```python
from build123d import *

# Parameters (mm, degrees)
SKETCH1_W             = 180
SKETCH1_H             = 180
BOSS_EXTRUDE1_DEPTH   = 3
FILLET1_R             = 15
SKETCH2_R             = 1.6
SKETCH2_W             = 25
SKETCH2_H             = 90
CUT_EXTRUDE2_DEPTH    = 128.314571044
FILLET2_R             = 10
HOLE_WIZARD_3_0_3_1_D = 3
HOLE_WIZARD_3_0_3_2_D = 3
HOLE_WIZARD_4_0_4_1_D = 4
SKETCH3_R             = 1.5
SKETCH3_R_2           = 1.6
CUT_EXTRUDE3_DEPTH    = 128.314571044
SKETCH4_R             = 1.5
CUT_EXTRUDE4_DEPTH    = 128.314571044
SKETCH5_R             = 12.5
CUT_EXTRUDE5_DEPTH    = 128.314571044
FILLET3_R             = 2


with BuildPart() as part:
    # Sketch1 → Boss-Extrude1 (new body)
    with BuildSketch(Plane(origin=(0, 0, 0), x_dir=(1, 0, 0), z_dir=(0, 1, 0))):
        Rectangle(SKETCH1_W, SKETCH1_H)
    extrude(amount=BOSS_EXTRUDE1_DEPTH)

    # Fillet1
    fillet1_edges = [part.edges().sort_by_distance(p)[0] for p in [
        (90, 1.5, 90),
        (-90, 1.5, 90),
        (-90, 1.5, -90),
        (90, 1.5, -90),
    ]]
    fillet(fillet1_edges, radius=FILLET1_R)

    # Sketch2 → Cut-Extrude2 (cut, through all)
    with BuildSketch(Plane(origin=(0, 3, 0), x_dir=(1, 0, 0), z_dir=(0, 1, 0))):
        with Locations(Location((-60.05, 20, 0), (0, 0, 270))):
            Circle(SKETCH2_R)
        with Locations(Location((-49.05, 20, 0), (0, 0, 270))):
            Circle(SKETCH2_R)
        with Locations(Location((-60.05, -20, 0), (0, 0, 270))):
            Circle(SKETCH2_R)
        with Locations(Location((-49.05, -20, 0), (0, 0, 270))):
            Circle(SKETCH2_R)
        with Locations(Location((49.05, 20, 0), (0, 0, 270))):
            Circle(SKETCH2_R)
        with Locations(Location((60.05, 20, 0), (0, 0, 270))):
            Circle(SKETCH2_R)
        with Locations(Location((49.05, -20, 0), (0, 0, 270))):
            Circle(SKETCH2_R)
        with Locations(Location((60.05, -20, 0), (0, 0, 270))):
            Circle(SKETCH2_R)
        with Locations((-77.5, 0)):
            Rectangle(SKETCH2_W, SKETCH2_H)
        with Locations((77.5, 0)):
            Rectangle(SKETCH2_W, SKETCH2_H)
    extrude(amount=-CUT_EXTRUDE2_DEPTH, mode=Mode.SUBTRACT)

    # Fillet2
    fillet2_edges = [part.edges().sort_by_distance(p)[0] for p in [
        (-65, 1.5, -45),
        (-65, 1.5, 45),
        (-90, 1.5, 45),
        (-90, 1.5, -45),
        (90, 1.5, -45),
        (90, 1.5, 45),
        (65, 1.5, 45),
        (65, 1.5, -45),
    ]]
    fillet(fillet2_edges, radius=FILLET2_R)

    # Диаметр отверстия Ø3.0 (3)1 (through all)
    with Locations(Plane(origin=(0, 3, 0), x_dir=(1, 0, 0), z_dir=(0, 1, 0))):
        with Locations((-65, -65), (-65, 65), (65, 65), (65, -65)):
            Hole(HOLE_WIZARD_3_0_3_1_D / 2)

    # Диаметр отверстия Ø3.0 (3)2 (through all)
    with Locations(Plane(origin=(0, 3, 0), x_dir=(1, 0, 0), z_dir=(0, 1, 0))):
        with Locations((-5, 15), (-38.5, 45.5), (-38.5, 55.5), (5, 15), (38.5, 45.5), (38.5, 55.5), (5, 86), (-5, 86)):
            Hole(HOLE_WIZARD_3_0_3_2_D / 2)

    # Диаметр отверстия Ø4.0 (4)1 (through all)
    with Locations(Plane(origin=(0, 3, 0), x_dir=(1, 0, 0), z_dir=(0, 1, 0))):
        with Locations((-19.5, 60), (19.5, 60)):
            Hole(HOLE_WIZARD_4_0_4_1_D / 2)

    # Sketch3 → Cut-Extrude3 (cut, through all)
    with BuildSketch(Plane(origin=(0, 3, 0), x_dir=(1, 0, 0), z_dir=(0, 1, 0))):
        with Locations(Location((-6, -72, 0), (0, 0, 270))):
            Circle(SKETCH3_R)
        with Locations(Location((6, -72, 0), (0, 0, 90))):
            Circle(SKETCH3_R)
        with Locations(Location((53.371589587, -44.65, 0), (0, 0, 270))):
            Circle(SKETCH3_R_2)
        with Locations(Location((-53.371589587, -44.65, 0), (0, 0, 270))):
            Circle(SKETCH3_R_2)
    extrude(amount=-CUT_EXTRUDE3_DEPTH, mode=Mode.SUBTRACT)

    # Sketch4 → Cut-Extrude4 (cut, through all)
    with BuildSketch(Plane(origin=(0, 3, 0), x_dir=(1, 0, 0), z_dir=(0, 1, 0))):
        with Locations(Location((-36, 83.5, 0), (0, 0, 270))):
            Circle(SKETCH4_R)
        with Locations(Location((37, 83.5, 0), (0, 0, 270))):
            Circle(SKETCH4_R)
        with Locations(Location((37, 26.5, 0), (0, 0, 270))):
            Circle(SKETCH4_R)
        with Locations(Location((-36, 26.5, 0), (0, 0, 270))):
            Circle(SKETCH4_R)
    extrude(amount=-CUT_EXTRUDE4_DEPTH, mode=Mode.SUBTRACT)

    # Sketch5 → Cut-Extrude5 (cut, through all)
    with BuildSketch(Plane(origin=(0, 3, 0), x_dir=(1, 0, 0), z_dir=(0, 1, 0))):
        with Locations(Location((0, 60, 0), (0, 0, 270))):
            Circle(SKETCH5_R)
        Polygon((31.754264805, 5), (0, -50), (-31.754264805, 5), (-24.826061575, 9), (0, -34), (24.826061575, 9), align=None)
        Polygon((0, -18), (15.588457268, 9), (-15.588457268, 9), align=None)
        Polygon((-5, -57.339745962), (-23.392304845, -57.339745962), (-45.598076211, -44.519237886), (-29, -15.770526581), align=None)
        Polygon((29, -15.770526581), (5, -57.339745962), (23.392304845, -57.339745962), (45.598076211, -44.519237886), align=None)
        with BuildLine():
            Line((-14.800549998, 50.996092632), (-27.5, 29))
            Line((-27.5, 29), (27.5, 29))
            Line((27.5, 29), (14.800549998, 50.996092632))
            Line((14.800549998, 50.996092632), (9.435897436, 47.078551181))
            ThreePointArc((9.435897436, 47.078551181), (0, 44), (-9.435897436, 47.078551181))
            Line((-9.435897436, 47.078551181), (-14.800549998, 50.996092632))
        make_face()
        Polygon((-59, -57.56624327), (-26.725386608, -76.2), (-59, -76.2), align=None)
        Polygon((-49.007586221, 49.3003268), (-32.726497308, 77.5), (-65.288675135, 77.5), align=None)
        Polygon((32.726497308, 77.5), (65.288675135, 77.5), (49.007586221, 49.3003268), align=None)
        Polygon((59, -57.56624327), (26.725386608, -76.2), (59, -76.2), align=None)
    extrude(amount=-CUT_EXTRUDE5_DEPTH, mode=Mode.SUBTRACT)

    # Fillet3
    fillet3_edges = [part.edges().sort_by_distance(p)[0] for p in [
        (0, 1.5, 18),
        (-15.588457268, 1.5, -9),
        (15.588457268, 1.5, -9),
        (-31.754264805, 1.5, -5),
        (-24.826061575, 1.5, -9),
        (0, 1.5, 34),
        (24.826061575, 1.5, -9),
        (31.754264805, 1.5, -5),
        (0, 1.5, 50),
        (-29, 1.5, 15.770526581),
        (-5, 1.5, 57.339745962),
        (-23.392304845, 1.5, 57.339745962),
        (-45.598076211, 1.5, 44.519237886),
        (29, 1.5, 15.770526581),
        (45.598076211, 1.5, 44.519237886),
        (23.392304845, 1.5, 57.339745962),
        (5, 1.5, 57.339745962),
        (27.5, 1.5, -29),
        (-27.5, 1.5, -29),
        (-14.800549998, 1.5, -50.996092632),
        (14.800549998, 1.5, -50.996092632),
        (-49.007586221, 1.5, -49.3003268),
        (-65.288675135, 1.5, -77.5),
        (-32.726497308, 1.5, -77.5),
        (49.007586221, 1.5, -49.3003268),
        (32.726497308, 1.5, -77.5),
        (65.288675135, 1.5, -77.5),
        (-59, 1.5, 76.2),
        (-59, 1.5, 57.56624327),
        (-26.725386608, 1.5, 76.2),
        (59, 1.5, 57.56624327),
        (59, 1.5, 76.2),
        (26.725386608, 1.5, 76.2),
    ]]
    fillet(fillet3_edges, radius=FILLET3_R)


solid = part.part
```
Geometry: final body of the model. Coordinates: model frame, mm. A direction names the side the tool comes from. Give positions to 0.01 mm unless a question says otherwise; leave off trailing zeros. Use one line per item in the form item = value.
Item 1: Line query: probe 1 along X at (y, z) = (2.3, 66); probe 2 along X at (y, z) = (2.25, -26); probe 3 along X at (y, z) = (0.7, 52). Output: solid intervals per line, ascending.
A:
probe_1 = -90 to -66.12, -63.88 to -59, -44.39 to 44.39, 59 to 63.88, 66.12 to 90
probe_2 = -65 to -37.41, -34.59 to 35.59, 38.41 to 65
probe_3 = -89.54 to -32.64, -8.08 to 8.08, 32.64 to 89.54
Item 2: Access query for faces 4 (the face through (67.85, 1.48, 41.99)), 5 (the face through (-57.24, 1.52, -63.56)), 6 (the face through (-68.01, 1.48, 42.15)), 7 (the face through (-85.72, 1.52, -85.49)). Directions: +Z, -Z, +X, -X, +Y, -Y. A direction counts if a zero-diameter tool reaches every point of the face in a straight line with its end or side. Return the directions, or none.
A:
face_4 = +X, +Y, -Y
face_5 = +Y, -Y
face_6 = -X, +Y, -Y
face_7 = -Z, -X, +Y, -Y
Item 3: Pin query (flat end, axial travel): P1, Ø1.5, axis at x = 78, y = 1.5, coming from the +Z side. Return the tip coordinate at first contact, or that it passes through.
A:
P1 = 89.83
Item 4: Section query A-A on y = 0.7. Give the number of separate pieces and of enclosed holes in the cut face, and give its area (3 significant figures).
A:
separate_pieces = 1
enclosed_holes = 40
area = 21,800 mm^2
Item 5: Draft query along X for faces 1 (the face through (87.15, 1.48, -48.01)), 2 (the face through (12.624, 1.521, 12.134)), 3 (the face through (-86.99, 1.48, -47.85)). Return one class per face: pulls with the +X half, pulls with the -X half, needs draft (parallel to the pull), parting line crosses it, or undercut.
A:
face_1 = pulls with the +X half
face_2 = undercut
face_3 = pulls with the -X half
